Geometry check sheet. Reference: drawing and pictorial views, mm from the part's lowest x, y, z. A direction names the side the tool comes from. Round coordinates to 2 decimals unless told otherwise and drop trailing zeros. Order: outer loops, then holes, each group sorted by start corner. A loop starts at its lowest first (then second) coordinate and runs counter-clockwise, first axis right, second up.
(1) Sectioned sample at C-C, the plane x = 46. Enter the section's corners in (y, z), and give its area (3 significant figures).
(2) Tool access check on the marked faces 1 and 2. Record the directions out of +Z, -Z, +X, -X, +Y, -Y that give a thin tool (end or side, any length) a straight path to the whole face; none if there is none.
(3) Thickness scan on probe 1 along Z at (x, y) = (27.5, 2.3); probe 2 along Y at (x, z) = (52, 19.5); probe 3 along X at (y, z) = (4, 27.5). Record the ranges inside material, lowest first.
(4) Sectioned sample at A-A, the plane z = 27.5. Enter the section's corners in (x, y), and give its area (3 significant figures).
(5) Sectioned sample at B-B, the plane x = 27.5. Enter the section's corners in (y, z).
(6) Depth check by flat-ended pin: pin 1 (2 mm diameter, centred on x = 48.5, z = 22, fed in from +Y); pin 2 (4 mm diameter, centred on x = 27.5, z = 51, fed in from +Y); pin 3 (4 mm diameter, centred on x = 38.5, y = 8, fed in from -Z); pin 4 (1.5 mm diameter, centred on x = 34, y = 12, fed in from +Z). Enter the tip coordinate at first touch or a pass-through.
(7) Sectioned sample at D-D, the plane y = 16. Enter the section's corners in (x, z).
(8) Mould release check, pull along Z, two halves, no side actions. Record for the marked faces 3, 4 and 5: released by +Z, released by -Z, zero draft, split by the parting line, or undercut.
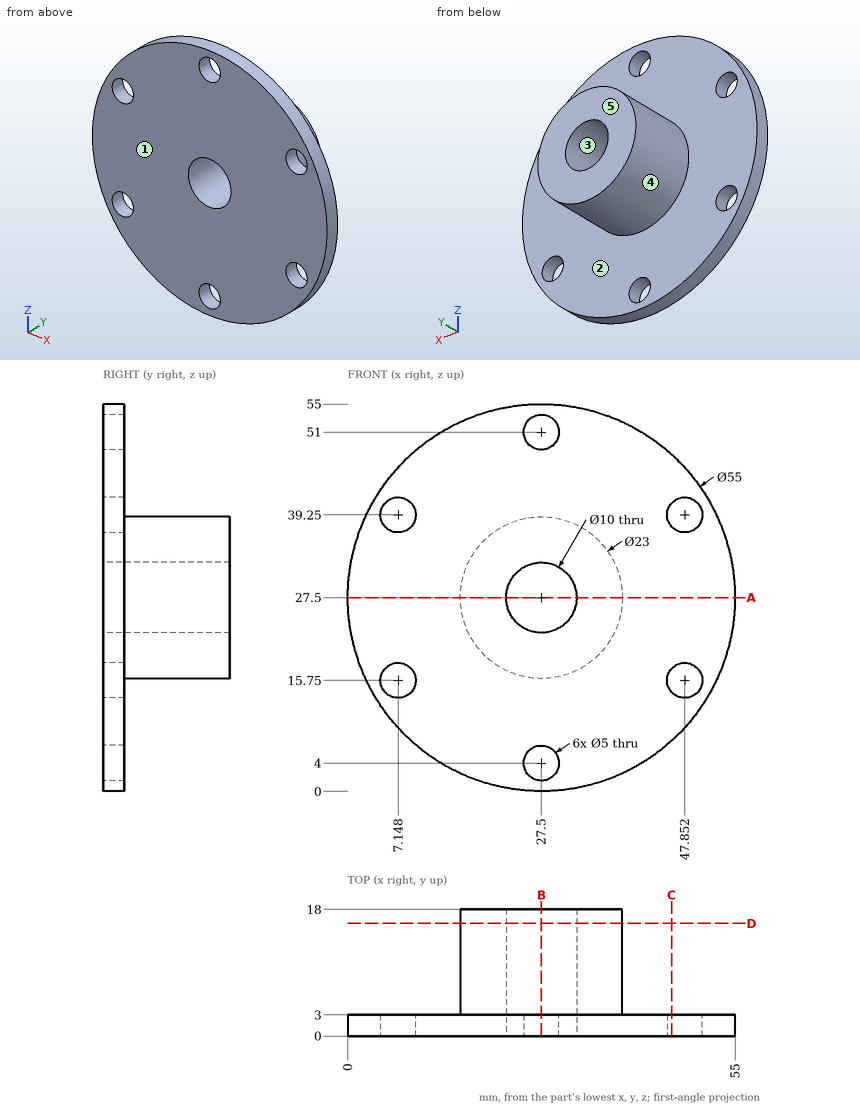
Derived:
1. outline: (0, 7.15) - (3, 7.15) - (3, 14.07) - (0, 14.07) - close; (0, 17.43) - (3, 17.43) - (3, 37.57) - (0, 37.57) - close; (0, 40.93) - (3, 40.93) - (3, 47.85) - (0, 47.85) - close
1. area: 102 mm2
2. face 1: +Z, -Z, +X, -X, -Y
2. face 2: +Y
3. probe 1: z = 0 to 1.5, 6.5 to 22.5, 32.5 to 48.5, 53.5 to 55
3. probe 2: y = 0 to 3
3. probe 3: x = 16 to 22.5, 32.5 to 39
4. outline: (0, 0) - (22.5, 0) - (22.5, 18) - (16, 18) - (16, 3) - (0, 3) - close; (32.5, 0) - (55, 0) - (55, 3) - (39, 3) - (39, 18) - (32.5, 18) - close
4. area: 330 mm2
5. outline: (0, 0) - (3, 0) - (3, 1.5) - (0, 1.5) - close; (0, 6.5) - (3, 6.5) - (3, 16) - (18, 16) - (18, 22.5) - (0, 22.5) - close; (0, 32.5) - (18, 32.5) - (18, 39) - (3, 39) - (3, 48.5) - (0, 48.5) - close; (0, 53.5) - (3, 53.5) - (3, 55) - (0, 55) - close
6. pin 1: stops at y = 3
6. pin 2: passes through
6. pin 3: stops at z = 20.34
6. pin 4: stops at z = 37.46
7. outline: circle Ø23 at (27.5, 27.5); hole circle Ø10 at (27.5, 27.5)
8. face 3: undercut
8. face 4: split by the parting line
8. face 5: zero draft
